Input: dimensioned drawing with shaded views. Units: mm. Origin: part minimum x, y, z. Coordinates: 2 decimals unless noted, no trailing zeros. Loops run counter-clockwise (first coordinate to the right, second up) from the corner with the lowest first, then second, coordinate; pieces in that order, holes last.
Item 1: Pin query (flat end, axial travel): pin 1 Ø1.9 at (x, y) = (2.81, 7.56) entering from -Z. Return the tip coordinate at first contact, or that it passes through.
Item 2: Line query: probe 1 along Y at (x, z) = (51, 1.45) (1 decimal); probe 2 along X at (y, z) = (39.5, 1.15) (1 decimal); probe 3 along X at (y, z) = (38, 0.8) (1 decimal). Output: solid intervals per line, ascending.
Item 3: Section query A-A, the plane x = 10. Return the cut outline in (y, z) (1 decimal).
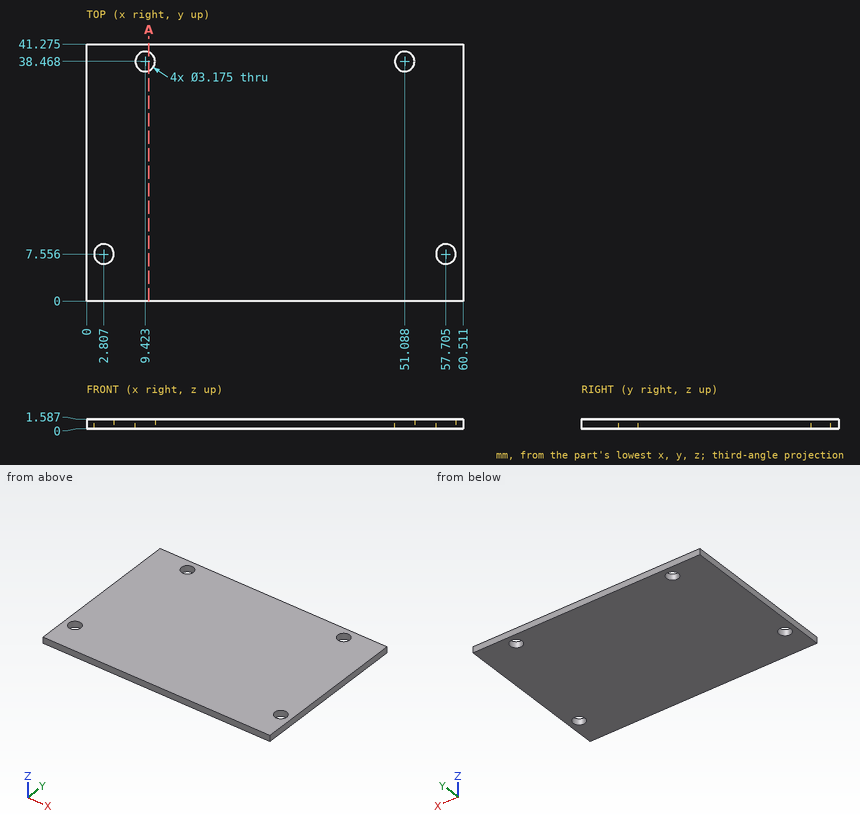
Verdict:
1. pin 1: passes through
2. probe 1: y = 0 to 36.9, 40.1 to 41.3
2. probe 2: x = 0 to 8.2, 10.6 to 49.9, 52.3 to 60.5
2. probe 3: x = 0 to 7.9, 10.9 to 49.6, 52.6 to 60.5
3. outline: (0, 0) - (37, 0) - (37, 1.6) - (0, 1.6) - close; (39.9, 0) - (41.3, 0) - (41.3, 1.6) - (39.9, 1.6) - close
